from build123d import *

# Parameters (mm, degrees)
F0_W     = 50.8
F0_H     = 25.4
F1_DEPTH = 76.2
F2_W     = 25.4
F2_H     = 38.1
F3_DEPTH = 19.05
F4_R     = 3.175
F5_DEPTH = 44.45
F6_R     = 3.175
F7_DEPTH = 76.2
F8_R     = 3.175
F9_DEPTH = 38.1
F10_R    = 5.08


with BuildPart() as f1:
    # F0 (on Front) → F1 (new body)
    with BuildSketch(Plane.XZ):
        with Locations((-25.4, 12.7)):
            Rectangle(F0_W, F0_H)
    extrude(amount=F1_DEPTH)

    # F2 (on face) → F3 (join)
    with BuildSketch(Plane.XY.offset(25.4)):
        with Locations((-25.4, -38.1)):
            Rectangle(F2_W, F2_H)
    extrude(amount=F3_DEPTH)

    # F4 (on face) → F5 (cut)
    with BuildSketch(Plane.XY.offset(44.45)):
        with Locations((-25.4, -28.575)):
            Circle(F4_R)
    extrude(amount=-F5_DEPTH, mode=Mode.SUBTRACT)

    # F6 (on face) → F7 (cut)
    with BuildSketch(Plane.XZ.offset(76.2)):
        with Locations((-25.4, 12.7)):
            Circle(F6_R)
    extrude(amount=-F7_DEPTH, mode=Mode.SUBTRACT)

    # F8 (on face) → F9 (cut)
    with BuildSketch(Plane.XZ.offset(57.15)):
        with Locations((-25.4, 34.925)):
            Circle(F8_R)
    extrude(amount=-F9_DEPTH, mode=Mode.SUBTRACT)

    # F10
    f10_edges = [f1.edges().sort_by_distance(p)[0] for p in [
        (-38.1, -38.1, 44.45),
        (-25.4, -19.05, 44.45),
        (-12.7, -38.1, 44.45),
        (-25.4, -57.15, 44.45),
        (-25.4, -19.05, 25.4),
        (-38.1, -38.1, 25.4),
        (-25.4, 0, 25.4),
        (0, 0, 12.7),
        (-25.4, 0, 0),
        (-50.8, 0, 12.7),
        (-50.8, -38.1, 25.4),
        (-50.8, -38.1, 0),
        (-50.8, -76.2, 12.7),
        (-25.4, -76.2, 25.4),
        (0, -38.1, 25.4),
    ]]
    fillet(f10_edges, radius=F10_R)


solid = f1.part
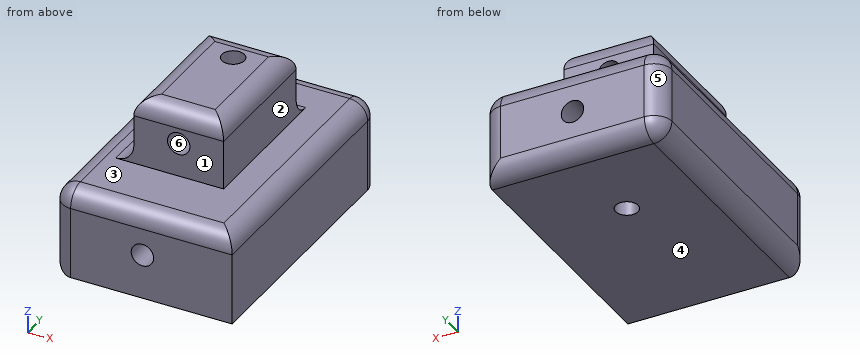
Here's how the part is built. I have some questions about the finished solid (model axes, mm). Face numbers are marked on the shaded views. A direction names the side the tool comes from. Give positions to 0.01 mm unless a question says otherwise; leave off trailing zeros. Order: outer loops, then holes, each group sorted by start corner. A loop starts at its lowest first (then second) coordinate and runs counter-clockwise, first axis right, second up. Notation, with made-up numbers: M 46,24 L 104,24 A24 cw 104,58 Z; hole C 33,47.5 d3. An arc over 180 degrees is marked long. Answer as a JSON object with one key per item and string values. Group by question number.
1) We'd pull the mould along Z, two halves only. Please class the marked faces 4, 5 and 6: pulls with the +Z half, pulls with the -Z half, needs draft (parallel to the pull), parting line crosses it, or undercut.
2) Please list where these lines run through material, in increasing order: L1, parallel to Z at x = -8, y = -65; L2, parallel to X at y = -29, z = 29.5; L3, parallel to Y at x = -13, z = 37. Write a range as [from, to].
3) Suppose I cut it at D-D, the plane x = -11.5. Write out the boundary of the cut face in (y, z), plus the area to 3 significant figures.
4) Suppose I cut it at A-A, the plane z = 36. Write out the boundary of the cut face in (x, y) (3 decimals), plus the area to 3 significant figures.
5) Suppose I cut it at C-C, the plane x = -25.4. Count the separate pieces of the cut face and the enclosed holes in it, plus the area to 3 significant figures.
6) I'm going to push flat-ended pins straight in: pin 1 Ø1.5 at (y, z) = (-41, 24.5) entering from -X; pin 2 Ø5.5 at (x, z) = (-25.4, 12.7) entering from -Y; pin 3 Ø6 at (x, y) = (-45.5, -10.5) entering from +Z; pin 4 Ø4 at (x, z) = (-29, 33.5) entering from -Y. Where does each tip first touch, or does it pass through?
7) Suppose I cut it at B-B, the plane y = -27.5. Write out the boundary of the cut face in (x, z) (3 decimals), plus the area to 3 significant figures.
8) On a 3-axis mill with a long thin cutter (end or side, diameter ignored), from which of +Z, -Z, +X, -X, +Y, -Y can I reach the whole of each face in a straight line? I mean the marked faces 1, 2 and 3. Say none if no direction works.
Results found:
{
 "1": {"face 4": "pulls with the -Z half", "face 5": "needs draft", "face 6": "undercut"},
 "2": {"L1": "[0, 25.4]", "L2": "[-38.2, -28.55], [-22.25, -12.7]", "L3": "[-57.15, -19.05]"},
 "3": {"outline": "M -76.2,0 L -5.08,0 A5.08 ccw 0,5.08 L 0,20.32 A5.08 ccw -5.08,25.4 L -71.12,25.4 A5.08 ccw -76.2,20.32 Z", "area": "1,920 mm²"},
 "4": {"outline": "M -38.1,-57.15 L -28.387,-57.15 L -28.387,-29.65 A3.175 cw -28.387,-27.5 L -28.387,-19.05 L -38.1,-19.05 Z; M -22.413,-57.15 L -12.7,-57.15 L -12.7,-19.05 L -22.413,-19.05 L -22.413,-27.5 A3.175 cw -22.413,-29.65 Z", "area": "740 mm²"},
 "5": {"separate pieces": "6", "enclosed holes": "0", "area": "1,710 mm²"},
 "6": {"pin 1": "x = -49.47", "pin 2": "through", "pin 3": "z = 25.4", "pin 4": "y = -57.15"},
 "7": {"outline": "M -50.8,5.08 A5.08 ccw -45.72,0 L -28.387,0 L -28.387,11.625 A3.175 cw -28.387,13.775 L -28.387,33.85 A3.175 cw -28.387,36 L -28.387,44.45 L -33.02,44.45 A5.08 ccw -38.1,39.37 L -38.1,30.48 A5.08 cw -43.18,25.4 L -45.72,25.4 A5.08 ccw -50.8,20.32 Z; M -22.413,0 L 0,0 L 0,20.32 A5.08 ccw -5.08,25.4 L -12.7,25.4 L -12.7,39.37 A5.08 ccw -17.78,44.45 L -22.413,44.45 L -22.413,36 A3.175 cw -22.413,33.85 L -22.413,13.775 A3.175 cw -22.413,11.625 Z", "area": "1,490 mm²"},
 "8": {"face 1": "+Z, +X, -X, -Y", "face 2": "+Z, +X, +Y, -Y", "face 3": "+Z"}
}
